Geometry: final body of the model. Coordinates: model frame, mm. Face numbers are marked on the shaded views. A direction names the side the tool comes from. Round coordinates to 2 decimals unless told otherwise and drop trailing zeros. Loops run counter-clockwise (first coordinate to the right, second up) from the corner with the lowest first, then second, coordinate; pieces in that order, holes last. Notation, with made-up numbers: M 7,38 L 17,38 A23 cw 17,58 Z; hole C 5.25,-16 d10. An arc over 180 degrees is marked long. Return JSON: item names as keys, results as strings.
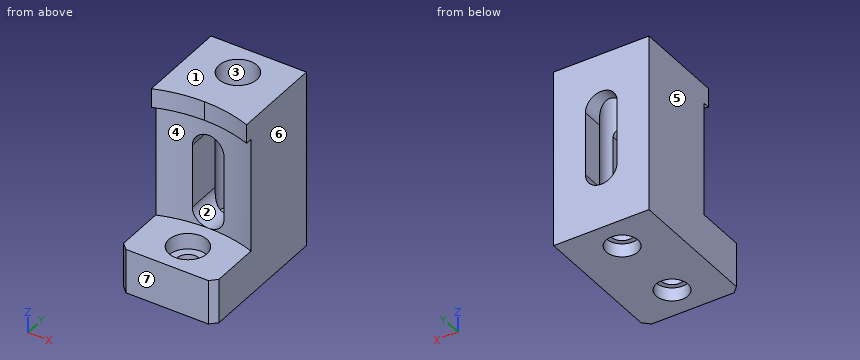
from build123d import *

# Parameters (mm, degrees)
F0_W      = 15
F0_H      = 22
F1_DEPTH  = 28
F3_DEPTH  = 3
F4_R      = 22.5
F5_DEPTH  = 18
F7_DEPTH  = 12.140320325
F8_R      = 2.5
F8_R_2    = 1.75
F9_DEPTH  = 2.1
F10_DEPTH = 7.7156429929
F11_R     = 3
F11_R_2   = 1.75
F12_DEPTH = 2.5
F13_R     = 3
F14_DEPTH = 23.5
F15_SIZE  = 1


with BuildPart() as f1:
    # F0 (on Top) → F1 (new body)
    with BuildSketch(Plane.XY):
        Rectangle(F0_W, F0_H)
    extrude(amount=F1_DEPTH)

    # F2 (on face) → F3 (cut)
    with BuildSketch(Plane.XY.offset(28)):
        with BuildLine():
            Line((-7.5, -11), (-7.5, -3.3505583204))
            ThreePointArc((-7.5, -3.3505583204), (-12.2678441464, -41.156443583), (21.5, -23.5))
            ThreePointArc((21.5, -23.5), (17.656443583, -11.2321558536), (7.5, -3.3505583204))
            Line((7.5, -3.3505583204), (7.5, -11))
            Line((7.5, -11), (-7.5, -11))
        make_face()
        with BuildLine():
            ThreePointArc((7.5, -3.3505583204), (3.8103152027, -2.3403332244), (0, -2))
            ThreePointArc((0, -2), (-3.8103152027, -2.3403332244), (-7.5, -3.3505583204))
            Line((-7.5, -3.3505583204), (-7.5, -11))
            Line((-7.5, -11), (7.5, -11))
            Line((7.5, -11), (7.5, -3.3505583204))
        make_face()
    extrude(amount=-F3_DEPTH, mode=Mode.SUBTRACT)

    # F4 (on face) → F5 (cut)
    with BuildSketch(Plane.XY.offset(25)):
        with Locations((0, -23.5)):
            Circle(F4_R)
    extrude(amount=-F5_DEPTH, mode=Mode.SUBTRACT)

    # F6 (on face) → F7 (cut, through all)
    with BuildSketch(Plane(origin=(0, 11, 0), x_dir=(-1, 0, 0), z_dir=(0, 1, 0))):
        with BuildLine():
            Line((-2.5, 19.5), (-2.5, 9.5))
            ThreePointArc((-2.5, 9.5), (0, 7), (2.5, 9.5))
            Line((2.5, 9.5), (2.5, 19.5))
            ThreePointArc((2.5, 19.5), (0, 22), (-2.5, 19.5))
        make_face()
    extrude(amount=-F7_DEPTH, mode=Mode.SUBTRACT)

    # F8 (on face) → F9 (cut)
    with BuildSketch(Plane(origin=(0, 0, 0), x_dir=(1, 0, 0), z_dir=(0, 0, -1))):
        with Locations((0, 6)):
            Circle(F8_R)
        with Locations((0, 6)):
            Circle(F8_R_2, mode=Mode.SUBTRACT)
        with Locations((0, -6)):
            Circle(F8_R)
        with Locations((0, -6)):
            Circle(F8_R_2, mode=Mode.SUBTRACT)
    extrude(amount=-F9_DEPTH, mode=Mode.SUBTRACT)

    # F10 (cut, through all): faces of the model
    f10_faces = [f1.faces().sort_by_distance(p)[0] for p in [
        (0, 6, 0),
        (0, -6, 0),
    ]]
    extrude(f10_faces, amount=-F10_DEPTH, mode=Mode.SUBTRACT)

    # F11 (on face) → F12 (cut)
    with BuildSketch(Plane.XY.offset(7)):
        with Locations((0, -6)):
            Circle(F11_R)
        with Locations((0, -6)):
            Circle(F11_R_2, mode=Mode.SUBTRACT)
    extrude(amount=-F12_DEPTH, mode=Mode.SUBTRACT)

    # F13 (on face) → F14 (cut)
    with BuildSketch(Plane.XY.offset(28)):
        with Locations((0, 6)):
            Circle(F13_R)
    extrude(amount=-F14_DEPTH, mode=Mode.SUBTRACT)

    # F15
    f15_edges = [f1.edges().sort_by_distance(p)[0] for p in [
        (7.5, -11, 3.5),
        (-7.5, -11, 3.5),
    ]]
    chamfer(f15_edges, length=F15_SIZE)


solid = f1.part
Q1. Section query D-D (z = 24.5). Output: boundary loops of the cut face in (x, y).
Determined:
{"outline": "M -7.5,-2.29 A22.5 cw 7.5,-2.29 L 7.5,11 L -7.5,11 Z; hole C 0,6 d6"}
Q2. Material intervals for L1, parallel to Y at x = 0, z = 1.15; L2, parallel to Y at x = 0, z = 5.6; L3, parallel to X at y = 8.25, z = 15, sorted ascending.
Determined:
{"L1": "y = -11 to -8.5, -3.5 to 3.5, 8.5 to 11", "L2": "y = -11 to -9, -3 to 3, 9 to 11", "L3": "x = -7.5 to -2.5, 2.5 to 7.5"}
Q3. Reachability of the marked faces 1, 2 and 3 from +Z, -Z, +X, -X, +Y, -Y: full face, straight path, thin tool, end or side. Return the list, or none.
Determined:
{"face 1": "+Z, +X, -X, +Y, -Y", "face 2": "+Y, -Y", "face 3": "+Z"}
Q4. Section query C-C (z = 12.25). Output: boundary loops of the cut face in (x, y).
Determined:
{"outline": "M -7.5,-2.29 A22.5 cw -2.5,-1.14 L -2.5,4.34 A3 cw -2.5,7.66 L -2.5,11 L -7.5,11 Z; M 2.5,-1.14 A22.5 cw 7.5,-2.29 L 7.5,11 L 2.5,11 L 2.5,7.66 A3 cw 2.5,4.34 Z"}
Q5. Pin query (flat end, axial travel): pin 1 (5 mm diameter, centred on x = 0, y = -6, fed in from +Z); pin 2 (1.5 mm diameter, centred on x = -1.5, z = 9.5, fed in from -Y); pin 3 (1.5 mm diameter, centred on x = -1, y = 7, fed in from -Z); pin 4 (5 mm diameter, centred on x = 3.5, z = 21.5, fed in from -Y). Return the tip coordinate at first contact, or that it passes through.
Determined:
{"pin 1": "stops at z = 4.5", "pin 2": "passes through", "pin 3": "stops at z = 2.1", "pin 4": "stops at y = -1.81"}
Q6. Pull-direction query (X, two-part tool) for the marked faces 4, 5, 6 and 7; classes: pulls with the +X half, pulls with the -X half, needs draft (parallel to the pull), parting line crosses it, or undercut.
Determined:
{"face 4": "undercut", "face 5": "pulls with the -X half", "face 6": "pulls with the +X half", "face 7": "needs draft"}
Q7. Section query A-A (y = -6). Output: boundary loops of the cut face in (x, z).
Determined:
{"outline": "M -7.5,0 L -2.5,0 L -2.5,2.1 L -1.75,2.1 L -1.75,4.5 L -3,4.5 L -3,7 L -7.5,7 Z; M 1.75,2.1 L 2.5,2.1 L 2.5,0 L 7.5,0 L 7.5,7 L 3,7 L 3,4.5 L 1.75,4.5 Z"}
Q8. Section query B-B (z = 2.75). Output: boundary loops of the cut face in (x, y), plus the area to 3 significant figures.
Determined:
{"outline": "M -7.5,-10 L -6.5,-11 L 6.5,-11 L 7.5,-10 L 7.5,11 L -7.5,11 Z; hole C 0,-6 d3.5; hole C 0,6 d3.5", "area": "310 mm^2"}
